```python
from build123d import *

# Parameters (mm, degrees)
BOSS_EXTRUDE3_DEPTH         = 50.8
F_1_4_0_25_DIAMETER_HOLE1_D = 6.35


with BuildPart() as part:
    # 3DSketch2 → Boss-Extrude3 (new, symmetric)
    with BuildSketch(Plane(origin=(69.85, 0, -9.525), x_dir=(-0.990830168044299, 0, 0.1351132047333135), z_dir=(0, -1, 0))):
        Polygon((0, 0), (33.031800727, 4.504336463), (33.306350759, 2.490969561), (38.025179435, 3.134446199), (37.750629402, 5.1478131), (55.053001212, 7.507227438), (55.327551244, 5.493860537), (60.046379919, 6.137337174), (59.771829887, 8.150704076), (138.418974476, 18.875314701), (140.992881026, 0), (2.57390655, -18.875314701), align=None)
    extrude(amount=BOSS_EXTRUDE3_DEPTH, both=True)

    # 1/4 (0.25) Diameter Hole1 (through all)
    with Locations(Plane(origin=(0, 0, -9.525), x_dir=(-1, 0, 0), z_dir=(0, 0, -1))):
        with Locations((60.325, -25.4), (60.325, 25.4)):
            Hole(F_1_4_0_25_DIAMETER_HOLE1_D / 2)


solid = part.part
```
Read the model definition and answer for the solid it produces. Units are mm, in the model's axes. A direction names the side the tool comes from. Give positions to 0.01 mm unless a question says otherwise; leave off trailing zeros. Order: outer loops, then holes, each group sorted by start corner. A loop starts at its lowest first (then second) coordinate and runs counter-clockwise, first axis right, second up. Notation, with made-up numbers: (-22.5, 8.5) -> (34.5, 8.5) arc R20 ccw to (34.5, 35.5) -> close; hole circle Ø2 at (27.25, 27). An arc over 180 degrees is marked (long way). Write item = value, one per line.
1. Given pin 1 (1.4 mm diameter, centred on x = 34, y = -17.5, fed in from -Z); pin 2 (5 mm diameter, centred on x = -60.325, y = 25.4, fed in from +Z), each flat-ended and moving along its own axis, determine where each tip first touches the part or whether it passes through.
Numbers:
pin_1 = -7.49
pin_2 = through
2. A cutting plane is placed at B-B, the plane x = -59.5. Write down the section's boundary in (y, z) (3 decimals), and give its area (3 significant figures).
Numbers:
outline = (-50.8, -9.525) -> (-28.466, -9.525) -> (-28.466, 9.525) -> (-50.8, 9.525) -> close; (-22.334, -9.525) -> (22.334, -9.525) -> (22.334, 9.525) -> (-22.334, 9.525) -> close; (28.466, -9.525) -> (50.8, -9.525) -> (50.8, 9.525) -> (28.466, 9.525) -> close
area = 1,700 mm²
3. The mould has two halves that part along Y. Classify faces 3 (the face through (-1, -50.8, 0)), 4 (the face through (-57.297, 26.354, 0.133)), 5 (the face through (12, -1, -7.493)), 6 (the face through (-1, 50.8, 0)): +Y half, -Y half, draft (parallel to the pull), parting line (faces both ways), or undercut.
Numbers:
face_3 = -Y half
face_4 = undercut
face_5 = draft
face_6 = +Y half
4. For faces 1 (the face through (34, -1, -7.493)), 2 (the face through (23, -1, -9.525)), determine the directions among +Z, -Z, +X, -X, +Y, -Y from which every point of the face is accessible in a straight line to the end or side of a thin tool.
Numbers:
face_1 = -Z, +Y, -Y
face_2 = -Z, +X, -X, +Y, -Y
